```python
from build123d import *

# Parameters (mm, degrees)
EXTRUDE_THIN1_DEPTH = 1.4
SKETCH2_W           = 10
SKETCH2_H           = 25
BOSS_EXTRUDE1_DEPTH = 4


with BuildPart() as part:
    # Sketch1 → Extrude-Thin1 (new body)
    with BuildSketch(Plane(origin=(0, 0, 0), x_dir=(1, 0, 0), z_dir=(0, 1, 0))):
        with BuildLine():
            Line((-2, 0), (-2, 49.1))
            ThreePointArc((-2, 49.1), (9.2, 60.3), (20.4, 49.1))
            Line((20.4, 49.1), (20.4, 0))
            ThreePointArc((20.4, 0), (9.2, -11.2), (-2, 0))
        make_face()
        with BuildLine():
            Line((0, 0), (0, 49.1))
            ThreePointArc((0, 49.1), (9.2, 58.3), (18.4, 49.1))
            Line((18.4, 49.1), (18.4, 0))
            ThreePointArc((18.4, 0), (9.2, -9.2), (0, 0))
        make_face(mode=Mode.SUBTRACT)
    extrude(amount=EXTRUDE_THIN1_DEPTH)

    # Sketch2 → Boss-Extrude1 (add)
    with BuildSketch(Plane.XZ):
        with BuildLine():
            Line((-2, 0), (-2, -49.1))
            ThreePointArc((-2, -49.1), (9.2, -60.3), (20.4, -49.1))
            Line((20.4, -49.1), (20.4, 0))
            ThreePointArc((20.4, 0), (9.2, 11.2), (-2, 0))
        make_face()
        with Locations((9.2, -24.55)):
            Rectangle(SKETCH2_W, SKETCH2_H, mode=Mode.SUBTRACT)
    extrude(amount=BOSS_EXTRUDE1_DEPTH)


solid = part.part
```
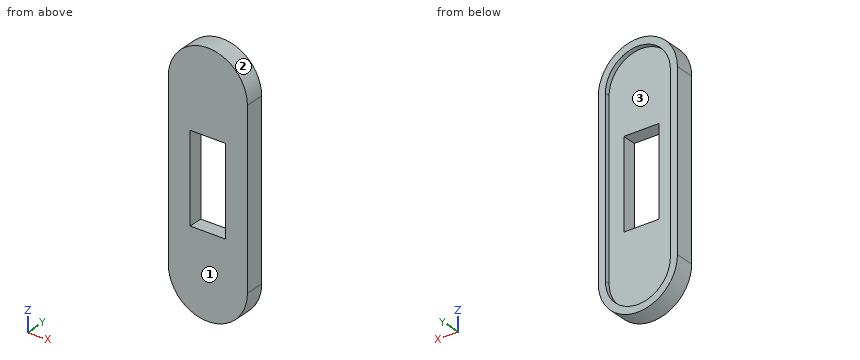
Check sheet for the modelled part. Datum: model origin and axes. Units: mm. Face numbers are marked on the shaded views. Give positions to 0.01 mm unless a question says otherwise; leave off trailing zeros. Write each loop counter-clockwise with the first axis right and the second up, starting at its lowest first coordinate (ties: lowest second). Pieces come first, ordered by that corner, then holes. Notation, with made-up numbers: (-32.5, -18.75) - (-2.5, -18.75) arc R12 ccw to (-2.5, -0.75) - close; hole circle Ø10 at (72.25, 84.25). An arc over 180 degrees is marked (long way). Answer as a JSON object with one key per item and string values. Group by question number.
1) Sectioned sample at B-B (y = -2.2). Record the cut outline in (x, z), then the cut area to 3 significant figures.
2) Sectioned sample at A-A (z = -32.5). Record the cut outline in (x, y).
3) Thickness scan on probe 1 along X at (y, z) = (0.8, -27); probe 2 along X at (y, z) = (-1.35, -32.5); probe 3 along Z at (x, y) = (13.5, -2.2). Record the ranges inside material, lowest first. Write a range as from..to.
4) Release check for a two-part mould opening along X. For the marked faces 1, 2 and 3 record: pulls with the +X half, pulls with the -X half, needs draft (parallel to the pull), parting line crosses it, or undercut.
5) Sectioned sample at D-D (z = -41). Record the cut outline in (x, y), then the cut area to 3 significant figures.
6) Depth check by flat-ended pin: P1, Ø2, axis at x = 7.5, y = -3, coming from the +Z side; P2, Ø8, axis at x = 13, z = -28, coming from the +Y side; P3, Ø2, axis at x = 11, z = -13.5, coming from the -Y side; P4, Ø1.2, axis at x = 7.5, y = -2, coming from the -Z side. Enter the tip coordinate at first touch or a pass-through.
7) Sectioned sample at C-C (x = 9.2). Record the cut outline in (y, z).
Geometry results:
{
 "1": {"outline": "(-2, -49.1) arc R11.2 ccw to (20.4, -49.1) - (20.4, 0) arc R11.2 ccw to (-2, 0) - close; hole (4.2, -37.05) - (14.2, -37.05) - (14.2, -12.05) - (4.2, -12.05) - close", "area": "1,240 mm^2"},
 "2": {"outline": "(-2, -4) - (4.2, -4) - (4.2, 0) - (0, 0) - (0, 1.4) - (-2, 1.4) - close; (14.2, -4) - (20.4, -4) - (20.4, 1.4) - (18.4, 1.4) - (18.4, 0) - (14.2, 0) - close"},
 "3": {"probe 1": "x = -2..0, 18.4..20.4", "probe 2": "x = -2..4.2, 14.2..20.4", "probe 3": "z = -59.44..-37.05, -12.05..10.34"},
 "4": {"face 1": "needs draft", "face 2": "parting line crosses it", "face 3": "undercut"},
 "5": {"outline": "(-2, -4) - (20.4, -4) - (20.4, 1.4) - (18.4, 1.4) - (18.4, 0) - (0, 0) - (0, 1.4) - (-2, 1.4) - close", "area": "95.2 mm^2"},
 "6": {"P1": "stops at z = 11.18", "P2": "stops at y = 0", "P3": "passes through", "P4": "stops at z = -60.25"},
 "7": {"outline": "(-4, -60.3) - (1.4, -60.3) - (1.4, -58.3) - (0, -58.3) - (0, -37.05) - (-4, -37.05) - close; (-4, -12.05) - (0, -12.05) - (0, 9.2) - (1.4, 9.2) - (1.4, 11.2) - (-4, 11.2) - close"}
}
